CAD build for the part. Positions are in the model's coordinates, mm. Face numbers are marked on the shaded views. A direction names the side the tool comes from. Give positions to 0.01 mm unless a question says otherwise; leave off trailing zeros. Write each loop counter-clockwise with the first axis right and the second up, starting at its lowest first coordinate (ties: lowest second). Pieces come first, ordered by that corner, then holes. Notation, with made-up numbers: (0.5, 10.5) - (32.5, 10.5) arc R22 cw to (32.5, 37.5) - close; hole circle Ø3 at (24.5, 4.25). An arc over 180 degrees is marked (long way). Put each result on its own line as item: value. Start each with the question number.
1. Drop flat-ended pins along their axis: pin 1 (1.5 mm diameter, centred on y = 30, z = 8.5, fed in from -X); pin 2 (1.5 mm diameter, centred on x = 26.5, z = 9.5, fed in from -Y); pin 3 (7.5 mm diameter, centred on y = 76, z = 8, fed in from -X). Give the stop position or say it passes through.
2. Mould opens along X. For the marked faces 1, 2, 3 and 4 say: +X half, -X half, draft (parallel to the pull), parting line (faces both ways), or undercut.
3. Cut at C-C on x = 69.5. List the corners of the cut face in (y, z), and give its area (3 significant figures).
4. Cut at A-A on y = 33. List the corners of the cut face in (x, z).
5. Wall check: line 1 (X direction, y = 65.5, z = 6); line 2 (Y direction, x = 75.5, z = 2); line 3 (X direction, y = 26, z = 7.25). Give the ranges that are in metal, low to high.
6. Tool access for the marked faces 5, 6 and 7: list every direction of +Z, -Z, +X, -X, +Y, -Y with a clear straight run to the whole face (end or side of a thin tool).
7. Cut at D-D on y = 73. List the corners of the cut face in (x, z).
8. Cut at B-B on z = 3.75. List the corners of the cut face in (x, y).
from build123d import *

# Parameters (mm, degrees)
F1_W     = 170
F1_H     = 80
F2_DEPTH = 15
F4_DEPTH = 15
F6_DEPTH = 25


with BuildPart() as f2:
    # F1 (on Top) → F2 (new body)
    with BuildSketch(Plane.XY):
        with Locations((0, 48.682307)):
            Rectangle(F1_W, F1_H)
    extrude(amount=F2_DEPTH)

    # F3 (on face) → F4 (cut)
    with BuildSketch(Plane.XY.offset(15)):
        Polygon((0, 64.682307), (-56, 8.682307), (56, 8.682307), align=None)
    extrude(amount=-F4_DEPTH, mode=Mode.SUBTRACT)

    # F5 (on face) → F6 (cut)
    with BuildSketch(Plane.XY.offset(15)):
        Polygon((-85, 88.682307), (-85, 27.037646), (-73, 27.037646), (-36.355339, 63.682307), (-36.355339, 88.682307), align=None)
        Polygon((85, 88.682307), (36.355339, 88.682307), (36.355339, 63.682307), (73, 27.037646), (85, 27.037646), align=None)
    extrude(amount=-F6_DEPTH, mode=Mode.SUBTRACT)


solid = f2.part
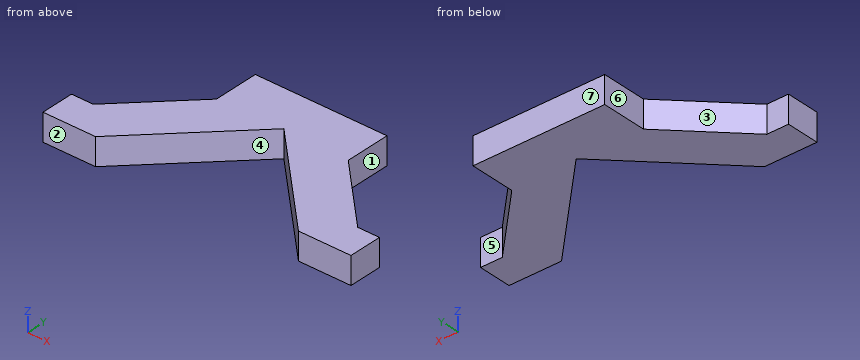
Report:
1. pin 1: stops at x = -70.79
1. pin 2: stops at y = 37.43
1. pin 3: stops at x = -36.36
2. face 1: +X half
2. face 2: draft
2. face 3: -X half
2. face 4: undercut
3. outline: (8.68, 0) - (30.54, 0) - (30.54, 15) - (8.68, 15) - close
3. area: 328 mm²
4. outline: (-67.04, 0) - (-31.68, 0) - (-31.68, 15) - (-67.04, 15) - close; (31.68, 0) - (67.04, 0) - (67.04, 15) - (31.68, 15) - close
5. line 1: x = -36.36 to 36.36
5. line 2: y = 8.68 to 27.04
5. line 3: x = -85 to -38.68, 38.68 to 85
6. face 5: +Z, -Z, +X, +Y
6. face 6: +Z, -Z, -X, +Y
6. face 7: +Z, -Z, +X, -X, +Y
7. outline: (-36.36, 0) - (36.36, 0) - (36.36, 15) - (-36.36, 15) - close
8. outline: (-85, 8.68) - (-56, 8.68) - (0, 64.68) - (56, 8.68) - (85, 8.68) - (85, 27.04) - (73, 27.04) - (36.36, 63.68) - (36.36, 88.68) - (-36.36, 88.68) - (-36.36, 63.68) - (-73, 27.04) - (-85, 27.04) - close
